For this review, take the finished solid that the model builds, in its own axes (mm). Face numbers are marked on the shaded views. A direction names the side the tool comes from. Round coordinates to 2 decimals unless told otherwise and drop trailing zeros. Order: outer loops, then holes, each group sorted by start corner. A loop starts at its lowest first (then second) coordinate and runs counter-clockwise, first axis right, second up. Notation, with made-up numbers: (33, 20) -> (72, 20) arc R28 cw to (72, 52) -> close; hole circle Ø10 at (7, 24.5). An arc over 180 degrees is marked (long way). Use a Markdown table: item, result. Add a question column.
1) Draft analysis for pull direction X (two halves, no side actions). For the marked faces 3, 4, 5 and 6, state which applies: pulls with the +X half, pulls with the -X half, needs draft (parallel to the pull), parting line crosses it, or undercut.
2) Consider section A-A (x = -10). State the section outline as (y, z) points.
3) Consider section D-D (y = 12.75). State the section outline as (x, z) points.
4) Machinability: for the marked faces 1 and 2, which of the approach directions +Z, -Z, +X, -X, +Y, -Y give a long, thin tool a straight path to every point of the face, cutting with its end or side? Answer none if there is none.
5) Consider section C-C (x = 24). State the section outline as (y, z) points, plus the area to 3 significant figures.
6) Clearance check with flat-ended pins moving along their axes: P1, Ø1.5, axis at x = -10.5, y = 12.5, coming from the -Z side; P2, Ø4.5, axis at x = -10, z = -48, coming from the +Y side; P3, Ø6, axis at y = 13.5, z = -11, coming from the +X side. State where each tip first meets the part, or that it passes through.
7) Wall thickness on line 1 along X through (y, z) = (2.5, -64); line 2 along X through (y, z) = (5.25, 10); line 3 along X through (y, z) = (14.75, -37.5): over which ranges is each line inside the solid? List them lowest first. Write a range as [from, to].
8) Consider section B-B (z = -10). State the section outline as (x, y) points, plus the area to 3 significant figures.
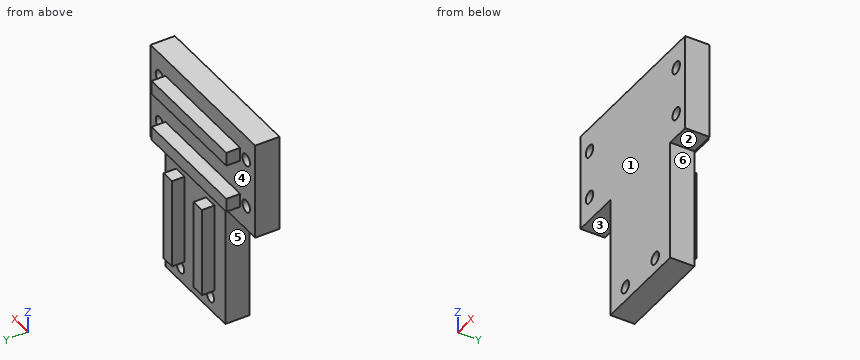
```python
from build123d import *

# Parameters (mm, degrees)
SALIENTE_EXTRUIR1_DEPTH = 10
SALIENTE_EXTRUIR3_DEPTH = 100
CROQUIS5_W              = 40
CROQUIS5_H              = 50
SALIENTE_EXTRUIR5_DEPTH = 10
SALIENTE_EXTRUIR7_DEPTH = 47
CROQUIS11_W             = 74.096638428
CROQUIS11_H             = 162.244793696
CORTAR_EXTRUIR3_DEPTH   = 30
CROQUIS9_W              = 10
CROQUIS9_H              = 40
CROQUIS9_W_2            = 40
CROQUIS9_H_2            = 10
CORTAR_EXTRUIR1_DEPTH   = 6.711119453
CROQUIS12_R             = 2.5
CORTAR_EXTRUIR4_DEPTH   = 11


with BuildPart() as part:
    # Croquis1 → Saliente-Extruir1 (new body)
    with BuildSketch(Plane(origin=(0, 0, 0), x_dir=(1, 0, 0), z_dir=(0, 1, 0))):
        Polygon((30, 20), (-30, 20), (-70, 20), (-70, -20), (-30, -20), (30, -20), align=None)
    extrude(amount=SALIENTE_EXTRUIR1_DEPTH)

    # Croquis3 → Saliente-Extruir3 (add, through all)
    with BuildSketch(Plane.ZY.offset(70)):
        Polygon((10, 10), (7.2, 10), (7.2, 15.711119453), (12.8, 15.711119453), (12.8, 10), align=None)
        Polygon((-10, 10), (-12.8, 10), (-12.8, 15.711119453), (-7.2, 15.711119453), (-7.2, 10), align=None)
    extrude(amount=-SALIENTE_EXTRUIR3_DEPTH)

    # Croquis5 → Saliente-Extruir5 (add)
    with BuildSketch(Plane(origin=(0, 10, 0), x_dir=(1, 0, 0), z_dir=(0, 1, 0))):
        with Locations((0, 45)):
            Rectangle(CROQUIS5_W, CROQUIS5_H)
    extrude(amount=-SALIENTE_EXTRUIR5_DEPTH)

    # Croquis7 → Saliente-Extruir7 (add)
    with BuildSketch(Plane(origin=(0, 0, -70), x_dir=(-1, 0, 0), z_dir=(0, 0, -1))):
        Polygon((12.8, 10), (10, 10), (7.2, 10), (7.2, 15.165648874), (12.8, 15.165648874), align=None)
        Polygon((-7.2, 10), (-10, 10), (-12.8, 10), (-12.8, 15.165648874), (-7.2, 15.165648874), align=None)
    extrude(amount=-SALIENTE_EXTRUIR7_DEPTH)

    # Croquis11 → Cortar-Extruir3 (cut)
    with BuildSketch(Plane.ZY.offset(70)):
        Rectangle(CROQUIS11_W, CROQUIS11_H)
    extrude(amount=-CORTAR_EXTRUIR3_DEPTH, mode=Mode.SUBTRACT)

    # Croquis9 → Cortar-Extruir1 (cut, through all)
    with BuildSketch(Plane(origin=(0, 10, 0), x_dir=(1, 0, 0), z_dir=(0, 1, 0))):
        with Locations((25, 0)):
            Rectangle(CROQUIS9_W, CROQUIS9_H)
        with Locations((0, 65)):
            Rectangle(CROQUIS9_W_2, CROQUIS9_H_2)
        with Locations((-35, 0)):
            Rectangle(CROQUIS9_W, CROQUIS9_H)
    extrude(amount=CORTAR_EXTRUIR1_DEPTH, mode=Mode.SUBTRACT)

    # Croquis12 → Cortar-Extruir4 (cut, through all)
    with BuildSketch(Plane(origin=(0, 10, 0), x_dir=(1, 0, 0), z_dir=(0, 1, 0))):
        with Locations((24, -10)):
            Circle(CROQUIS12_R)
        with Locations((24, 10)):
            Circle(CROQUIS12_R)
        with Locations((-34, -10)):
            Circle(CROQUIS12_R)
        with Locations((-34, 10)):
            Circle(CROQUIS12_R)
        with Locations((10, 64)):
            Circle(CROQUIS12_R)
        with Locations((-10, 64)):
            Circle(CROQUIS12_R)
    extrude(amount=-CORTAR_EXTRUIR4_DEPTH, mode=Mode.SUBTRACT)


solid = part.part
```
Results list:
| question | item | result |
|---|---|---|
| 1 | face 3 | needs draft |
| 1 | face 4 | undercut |
| 1 | face 5 | pulls with the -X half |
| 1 | face 6 | pulls with the +X half |
| 2 | outline | (0, -70) -> (10, -70) -> (10, -66.5) -> (0, -66.5) -> close; (0, -61.5) -> (10, -61.5) -> (10, -60) -> (15.17, -60) -> (15.17, -23) -> (10, -23) -> (10, -12.8) -> (15.71, -12.8) -> (15.71, -7.2) -> (10, -7.2) -> (10, 7.2) -> (15.71, 7.2) -> (15.71, 12.8) -> (10, 12.8) -> (10, 20) -> (0, 20) -> close |
| 3 | outline | (-30, -12.8) -> (20, -12.8) -> (20, -7.2) -> (-30, -7.2) -> close; (-30, 7.2) -> (20, 7.2) -> (20, 12.8) -> (-30, 12.8) -> close; (-12.8, -60) -> (-7.2, -60) -> (-7.2, -23) -> (-12.8, -23) -> close; (7.2, -60) -> (12.8, -60) -> (12.8, -23) -> (7.2, -23) -> close |
| 4 | face 1 | +Z, -Z, +X, -X, -Y |
| 4 | face 2 | -Z, +X, +Y, -Y |
| 5 | outline | (0, -20) -> (10, -20) -> (10, -12.5) -> (0, -12.5) -> close; (0, -7.5) -> (10, -7.5) -> (10, 7.5) -> (0, 7.5) -> close; (0, 12.5) -> (10, 12.5) -> (10, 20) -> (0, 20) -> close |
| 5 | area | 300 mm2 |
| 6 | P1 | z = -60 |
| 6 | P2 | y = 15.17 |
| 6 | P3 | x = 20 |
| 7 | line 1 | [-20, -12.5], [-7.5, 7.5], [12.5, 20] |
| 7 | line 2 | [-40, -36.5], [-31.5, 21.5], [26.5, 30] |
| 7 | line 3 | [-12.8, -7.2], [7.2, 12.8] |
| 8 | outline | (-40, 0) -> (-36.5, 0) -> (-36.5, 10) -> (-40, 10) -> close; (-31.5, 0) -> (21.5, 0) -> (21.5, 10) -> (20, 10) -> (20, 15.71) -> (-30, 15.71) -> (-30, 10) -> (-31.5, 10) -> close; (26.5, 0) -> (30, 0) -> (30, 10) -> (26.5, 10) -> close |
| 8 | area | 886 mm2 |
